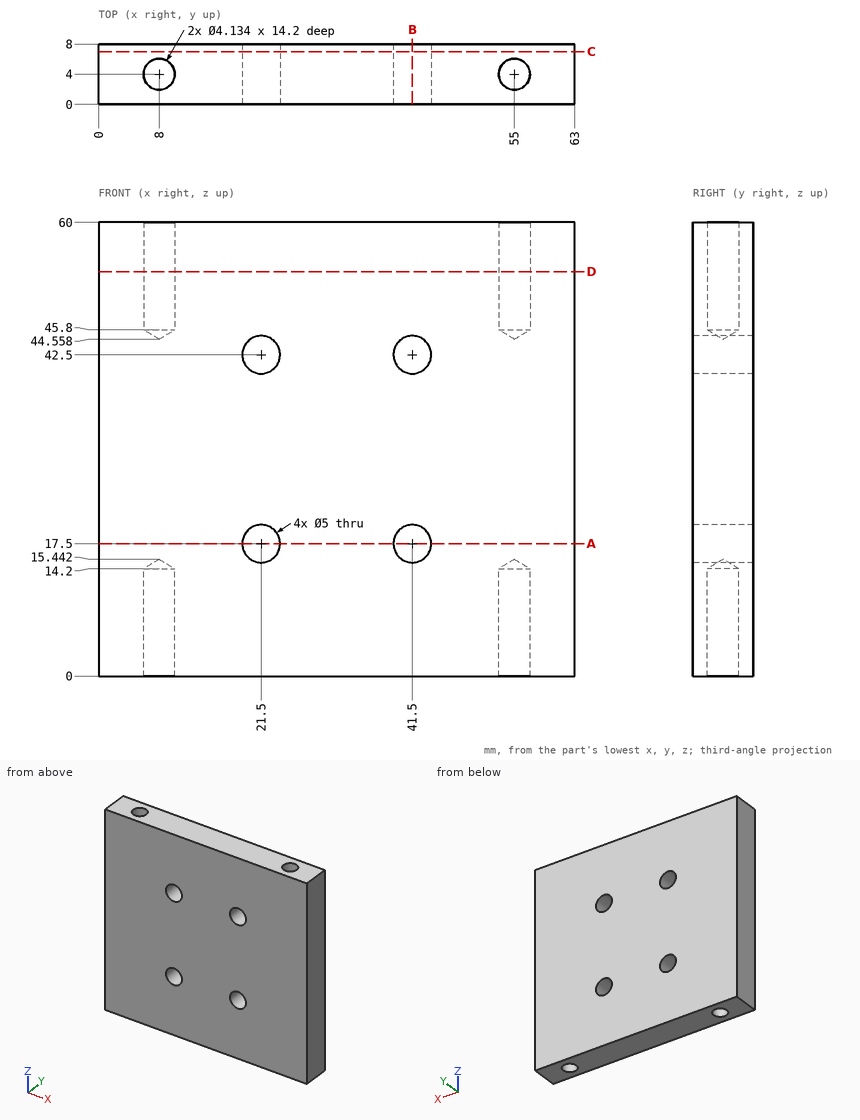
For this review, use the dimensioned drawing (mm, ordinates from the lowest corner) and the shaded views. Give positions to 0.01 mm unless a question says otherwise; leave off trailing zeros. Order: outer loops, then holes, each group sorted by start corner. A loop starts at its lowest first (then second) coordinate and runs counter-clockwise, first axis right, second up. Notation, with made-up numbers: (-4.75, -40) - (47.25, -40) arc R16 ccw to (47.25, -21) - close; hole circle Ø9 at (14.5, -12). An arc over 180 degrees is marked (long way). Use CSV: the item, a comma, the result in double quotes. Start each with the question number.
Q1. For P1, Ø3.5, axis at x = 8, y = 4, coming from the -Z side; P2, Ø3.5, axis at x = 55, y = 4, coming from the +Z side, all flat-tipped, find the tip position at first contact; note any pin that passes through.
Q2. Take a section at C-C (y = 7). State the section outline as (x, z) points, and give its area (3 significant figures).
Q3. Take a section at B-B (x = 41.5). State the section outline as (y, z) points.
Q4. Take a section at A-A (z = 17.5). State the section outline as (x, y) points, and give its area (3 significant figures).
Q5. Take a section at D-D (z = 53.5). State the section outline as (x, y) points, and give its area (3 significant figures).
Q6. For line 1 (X direction, y = 4, z = 42.5); line 2 (X direction, y = 4, z = 56.75); line 3 (Z direction, x = 41.5, y = 5), list the stretches that pass through material, from the lowest coordinate up.
Calculated:
1,P1,"stops at z = 14.39"
1,P2,"stops at z = 45.61"
2,outline,"(0, 0) - (63, 0) - (63, 60) - (0, 60) - close; hole circle Ø5 at (21.5, 17.5); hole circle Ø5 at (21.5, 42.5); hole circle Ø5 at (41.5, 17.5); hole circle Ø5 at (41.5, 42.5)"
2,area,"3,700 mm²"
3,outline,"(0, 0) - (8, 0) - (8, 15) - (0, 15) - close; (0, 20) - (8, 20) - (8, 40) - (0, 40) - close; (0, 45) - (8, 45) - (8, 60) - (0, 60) - close"
4,outline,"(0, 0) - (19, 0) - (19, 8) - (0, 8) - close; (24, 0) - (39, 0) - (39, 8) - (24, 8) - close; (44, 0) - (63, 0) - (63, 8) - (44, 8) - close"
4,area,"424 mm²"
5,outline,"(0, 0) - (63, 0) - (63, 8) - (0, 8) - close; hole circle Ø4.13 at (8, 4); hole circle Ø4.13 at (55, 4)"
5,area,"477 mm²"
6,line 1,"x = 0 to 19, 24 to 39, 44 to 63"
6,line 2,"x = 0 to 5.93, 10.07 to 52.93, 57.07 to 63"
6,line 3,"z = 0 to 15, 20 to 40, 45 to 60"
